Work out the finished part from the listing and answer in its coordinate system (mm). A direction names the side the tool comes from. Round coordinates to 2 decimals unless told otherwise and drop trailing zeros. Loops run counter-clockwise (first coordinate to the right, second up) from the corner with the lowest first, then second, coordinate; pieces in that order, holes last. Notation, with made-up numbers: (-22, -28) - (33, -28) arc R10 ccw to (33, -17) - close; hole circle Ø9 at (-6.75, 57). An arc over 180 degrees is marked (long way). Return JSON: item names as keys, results as strings.
from build123d import *

# Parameters (mm, degrees)
F0_R     = 200
F1_DEPTH = 800
F2_SIZE2 = 200
F2_SIZE  = 697.4828887682
F3_R     = 145
F4_DEPTH = 40


with BuildPart() as f1:
    # F0 (on Top) → F1 (new body)
    with BuildSketch(Plane.XY):
        Circle(F0_R)
    extrude(amount=F1_DEPTH)

    # F2
    f2_edges = [f1.edges().sort_by_distance(p)[0] for p in [
        (-200, 0, 800),
    ]]
    f2_side = f1.faces().sort_by_distance((-200, 0, 400))[0]
    chamfer(f2_edges, length=F2_SIZE, length2=F2_SIZE2, reference=f2_side)

    # F3 (on face) → F4 (join)
    with BuildSketch(Plane(origin=(0, 0, 0), x_dir=(1, 0, 0), z_dir=(0, 0, -1))):
        Circle(F3_R)
    extrude(amount=F4_DEPTH)


solid = f1.part
1) A tool of negligible diameter and unlimited length cuts with its end or side. For faces 1 (the cylindrical face through (190.764, 60.075, 50.541)), 2 (the flat face through (132.4, 60.2, 0)), from which of +Z, -Z, +X, -X, +Y, -Y can it reach the whole face along a straight path? Write none if from no direction.
Verdict:
{"face 1": "+Z, -Z", "face 2": "-Z"}
2) Flat-ended cylindrical pins translate along their axes: pin 1 (1.5 mm diameter, centred on x = 90.5, z = 449, fed in from -Y); pin 2 (1 mm diameter, centred on y = -21.5, z = 308, fed in from +X); pin 3 (2 mm diameter, centred on x = 80, z = 406, fed in from +Y). Find the tip coordinate at first contact, or state that the pin passes through.
Verdict:
{"pin 1": "stops at y = -45.63", "pin 2": "stops at x = 139.59", "pin 3": "stops at y = 80.84"}
3) Section A-A (z = 711) is taken. Give the vertices of the cut face in (x, y), and give its area (3 significant figures).
Verdict:
{"outline": "circle Ø51.04 at (0, 0)", "area": "2,050 mm2"}
4) Find the intervals of material crossed by L1, parallel to Y at x = -176, z = 32; L2, parallel to X at y = 124.5, z = 20.5; L3, parallel to Y at x = -58, z = 208.5, in increasing order.
Verdict:
{"L1": "y = -94.99 to 94.99", "L2": "x = -156.52 to 156.52", "L3": "y = -159.38 to 159.38"}
5) Section B-B (z = 256.5) is taken. Give the vertices of the cut face in (x, y).
Verdict:
{"outline": "circle Ø311.69 at (0, 0)"}
